For this review, take the finished solid that the model builds, in its own axes (mm). A direction names the side the tool comes from. Give positions to 0.01 mm unless a question says otherwise; leave off trailing zeros. Write each loop counter-clockwise with the first axis right and the second up, starting at its lowest first coordinate (ties: lowest second). Pieces come first, ordered by that corner, then holes.
Q1. We need section A-A (z = 1.9). Give the number of separate pieces and of enclosed holes in the cut face, then the cut area to 3 significant figures.
Q2. We need section B-B (y = -21). Write out the cut boundary in (x, z).
Q3. Insertion check: P1, Ø1.5, axis at x = -26.5, z = 1, coming from the -Y side; P2, Ø1.5, axis at x = -35, z = 1.5, coming from the -Y side. Each pin has a flat end and moves straight along its axis. Give the tip position at first contact, or say it passes through.
Q4. For line 1 (X direction, y = 148, z = 2.3) (3 decimals); line 2 (X direction, y = 38, z = 2.65); line 3 (Y direction, x = 39, z = 2.4) (3 decimals), list the stretches that pass through material, from the lowest coordinate up.
Q5. Machinability: for faces 1 (the flat face through (-39.202, 15.998, 1.479)), 2 (the flat face through (-1, 57, 3)), which of the approach directions +Z, -Z, +X, -X, +Y, -Y give a long, thin tool a straight path to every point of the face, cutting with its end or side? Answer none if there is none.
Q6. Mouldability with a two-part tool opening along Y and no side actions: class faces 3 (the flat face through (38.948, 15.722, 1.479)), 4 (the cylindrical face through (-43.168, -35.185, 1.479)), 5 (the cylindrical face through (32, -21.9, 1.5)), 6 (the cylindrical face through (48, 153.9, 1.5)) as released by +Y, released by -Y, zero draft, split by the parting line, or undercut.
```python
from build123d import *

# Parameters (mm, degrees)
SKETCH1_W           = 9.2
SKETCH1_H           = 14.65
SKETCH1_R           = 1.575
SKETCH1_W_2         = 10
SKETCH1_H_2         = 5
SKETCH1_W_3         = 3.15
SKETCH1_H_3         = 20
SKETCH1_H_4         = 12
BOSS_EXTRUDE2_DEPTH = 3
FILLET1_R           = 7


with BuildPart() as part:
    # Sketch1 → Boss-Extrude2 (new body)
    with BuildSketch(Plane.XY):
        with BuildLine():
            Line((-30, -39), (30, -39))
            ThreePointArc((30, -39), (42.910893348, -35.38119113), (50, -24))
            Line((50, -24), (30, -24))
            Line((30, -24), (30, 6))
            Line((30, 6), (50, 27.730066792))
            Line((50, 27.730066792), (50, 101.943914812))
            Line((50, 101.943914812), (48.6, 101.943914812))
            Line((48.6, 101.943914812), (48.6, 113.943914812))
            Line((48.6, 113.943914812), (50, 113.943914812))
            Line((50, 113.943914812), (50, 156))
            Line((50, 156), (-50, 156))
            Line((-50, 156), (-50, 113.943914812))
            Line((-50, 113.943914812), (-48.6, 113.943914812))
            Line((-48.6, 113.943914812), (-48.6, 101.943914812))
            Line((-48.6, 101.943914812), (-50, 101.943914812))
            Line((-50, 101.943914812), (-50, 27.730066792))
            Line((-50, 27.730066792), (-30, 6))
            Line((-30, 6), (-30, -24))
            Line((-30, -24), (-50, -24))
            ThreePointArc((-50, -24), (-42.910893348, -35.38119113), (-30, -39))
        make_face()
        with Locations((-35.4, 33.675)):
            Rectangle(SKETCH1_W, SKETCH1_H, mode=Mode.SUBTRACT)
        with Locations((0, -27)):
            Circle(SKETCH1_R, mode=Mode.SUBTRACT)
        with Locations((22.5, -9)):
            Circle(SKETCH1_R, mode=Mode.SUBTRACT)
        with Locations((-22.5, -9)):
            Circle(SKETCH1_R, mode=Mode.SUBTRACT)
        with Locations((0, -9)):
            Rectangle(SKETCH1_W_2, SKETCH1_H_2, mode=Mode.SUBTRACT)
        with Locations((39, 148)):
            Circle(SKETCH1_R, mode=Mode.SUBTRACT)
        with Locations((-39, 62)):
            Circle(SKETCH1_R, mode=Mode.SUBTRACT)
        with Locations((-19.246461744, 100.75)):
            Rectangle(SKETCH1_W_3, SKETCH1_H_3, mode=Mode.SUBTRACT)
        with Locations((-28.425, 107.943914812)):
            Rectangle(SKETCH1_W_3, SKETCH1_H_4, mode=Mode.SUBTRACT)
        with Locations((-39, 148)):
            Circle(SKETCH1_R, mode=Mode.SUBTRACT)
        with Locations((19.246461744, 100.75)):
            Rectangle(SKETCH1_W_3, SKETCH1_H_3, mode=Mode.SUBTRACT)
        with Locations((39, 62)):
            Circle(SKETCH1_R, mode=Mode.SUBTRACT)
        with Locations((28.425, 107.943914812)):
            Rectangle(SKETCH1_W_3, SKETCH1_H_4, mode=Mode.SUBTRACT)
    extrude(amount=BOSS_EXTRUDE2_DEPTH)

    # Fillet1
    # the kernel refuses this fillet: 7 mm, written as the material it adds along each edge
    with BuildSketch(Plane(origin=(-30, -39, 0), x_dir=(1, 0, 0), z_dir=(0, 0, 1))) as fillet1_piece_1:
        with BuildLine():
            CenterArc((0.312366932, -7), FILLET1_R, 90, 4.731570596)
            ThreePointArc((-0.265046647, -0.023855394), (-0.132480496, -0.012403535), (0, 0))
            Line((0, 0), (0.312366932, 0))
        make_face()
    extrude(amount=3)
    with BuildSketch(Plane(origin=(-30, -24, 0), x_dir=(0, 1, 0), z_dir=(0, 0, 1)), Plane(origin=(30, -24, 0), x_dir=(1, 0, 0), z_dir=(0, 0, 1))) as fillet1_piece_2:
        with BuildLine():
            CenterArc((FILLET1_R, FILLET1_R), FILLET1_R, 180, 90)
            Line((0, FILLET1_R), (0, 0))
            Line((0, 0), (FILLET1_R, 0))
        make_face()
    extrude(amount=3)
    with BuildSketch(Plane(origin=(30, -39, 0), x_dir=(-1, 0, 0), z_dir=(0, 0, 1))) as fillet1_piece_3:
        with BuildLine():
            CenterArc((0.312366932, 7), FILLET1_R, 265.268429404, 4.731570596)
            ThreePointArc((-0.265046647, 0.023855394), (-0.132480496, 0.012403535), (0, 0))
            Line((0, 0), (0.312366932, 0))
        make_face()
    extrude(amount=3)
    # the kernel refuses this fillet: 7 mm, written as the material it takes off along each edge
    with BuildSketch(Plane(origin=(-50, 27.730066792, -6.827532689), x_dir=(0, 1, 0), z_dir=(0, 0, 1)), Plane(origin=(50, 27.730066792, -6.827532689), x_dir=(-0.6772094339211744, -0.7357903115753581, 0), z_dir=(0, 0, 1))) as fillet1_2_piece_1:
        with BuildLine():
            CenterArc((FILLET1_R * 0.390144725089, -FILLET1_R), FILLET1_R, 90, 42.625961352)
            Line((-FILLET1_R * 0.287064708832, -FILLET1_R * 0.264209688425), (0, 0))
            Line((0, 0), (FILLET1_R * 0.390144725089, 0))
        make_face()
    extrude(amount=16.655065378, mode=Mode.SUBTRACT)
    with BuildSketch(Plane(origin=(-50, 156, -17.5), x_dir=(1, 0, 0), z_dir=(0, 0, 1)), Plane(origin=(50, 156, -17.5), x_dir=(0, -1, 0), z_dir=(0, 0, 1))) as fillet1_2_piece_2:
        with BuildLine():
            CenterArc((FILLET1_R, -FILLET1_R), FILLET1_R, 90, 90)
            Line((0, -FILLET1_R), (0, 0))
            Line((0, 0), (FILLET1_R, 0))
        make_face()
    extrude(amount=38, mode=Mode.SUBTRACT)


solid = part.part
```
Computed:
1. separate pieces: 1
1. enclosed holes: 13
1. area: 17,300 mm2
2. outline: (-31.26, 0) - (31.26, 0) - (31.26, 3) - (-31.26, 3) - close
3. P1: stops at y = -39
3. P2: stops at y = -38.92
4. line 1: x = -50 to -40.575, -37.425 to 37.425, 40.575 to 50
4. line 2: x = -50 to -40, -30.8 to 50
4. line 3: y = -37.628 to -24, 15.779 to 60.425, 63.575 to 146.425, 149.575 to 156
5. face 1: +Z, -Z, -X
5. face 2: +Z, +X, -X, +Y, -Y
6. face 3: undercut
6. face 4: released by -Y
6. face 5: undercut
6. face 6: released by +Y
